Source: CAD feature listing. Evaluate the final solid. Frame: model axes, mm. Give positions to 0.01 mm unless a question says otherwise; leave off trailing zeros. Write each question's results on one line, items separated by ' | '. Start each with the question number.
Item 1: Contact query for a flat-ended pin moving along its axis: pin 1 Ø13 at (x, y) = (-143.58, -131.25) entering from +Z. Output: stop coordinate, or through.
Item 2: Line query: line 1 along X through (y, z) = (-92, 4.15); line 2 along X through (y, z) = (-92.5, 3.6); line 3 along Y through (x, z) = (-215, 0.3). Output: solid intervals per line, ascending.
Item 3: Mould query, pull axis X, two halves, no side actions, for faces 1 (the flat face through (-223.011, -76, 2)), 2 (the cylindrical face through (-189.42, -128.54, 2.54)), 3 (the flat face through (-174, -73, 0)). Classes: released by +X, released by -X, zero draft, split by the parting line, or undercut.
Item 4: Section A-A on z = 3.9. State how many separate pieces and enclosed holes the cut face has, and give its area (3 significant figures).
```python
from build123d import *

# Parameters (mm, degrees)
SKETCH2_W           = 100
SKETCH2_H           = 150
BOSS_EXTRUDE1_DEPTH = 5
SKETCH3_R           = 4.1021
CUT_EXTRUDE1_DEPTH  = 5
SKETCH6_R           = 3.2639
CUT_EXTRUDE2_DEPTH  = 269.528430204


with BuildPart() as part:
    # Sketch2 → Boss-Extrude1 (new body)
    with BuildSketch(Plane.XY):
        with Locations((-173.010889244, -74.49468588)):
            Rectangle(SKETCH2_W, SKETCH2_H)
    extrude(amount=BOSS_EXTRUDE1_DEPTH)

    # Sketch3 → Cut-Extrude1 (cut)
    with BuildSketch(Plane(origin=(0, 0, 0), x_dir=(-1, 0, 0), z_dir=(0, 0, -1))):
        with Locations((212.756022811, -54.012878845)):
            Circle(SKETCH3_R)
        with Locations((212.756022811, -94.012878845)):
            Circle(SKETCH3_R)
        with Locations((143.584758496, -18.75)):
            Circle(SKETCH3_R)
        with Locations((143.584758496, -56.25)):
            Circle(SKETCH3_R)
        with Locations((143.584758496, -93.75)):
            Circle(SKETCH3_R)
        with Locations((143.584758496, -131.25)):
            Circle(SKETCH3_R)
    extrude(amount=-CUT_EXTRUDE1_DEPTH, mode=Mode.SUBTRACT)

    # Sketch6 → Cut-Extrude2 (cut, through all)
    with BuildSketch(Plane.XY.offset(5)):
        with Locations((-187.010889244, -18.24468588)):
            Circle(SKETCH6_R)
        with Locations((-187.010889244, -55.74468588)):
            Circle(SKETCH6_R)
        with Locations((-187.010889244, -93.24468588)):
            Circle(SKETCH6_R)
        with Locations((-187.010889244, -130.74468588)):
            Circle(SKETCH6_R)
    extrude(amount=-CUT_EXTRUDE2_DEPTH, mode=Mode.SUBTRACT)


solid = part.part
```
Evaluation:
1) pin 1: stops at z = 5
2) line 1: x = -223.01 to -216.33, -209.18 to -190.03, -183.99 to -147.29, -139.87 to -123.01 | line 2: x = -223.01 to -216.57, -208.94 to -190.19, -183.83 to -147.49, -139.68 to -123.01 | line 3: y = -149.49 to -97.45, -90.58 to -57.45, -50.58 to 0.51
3) face 1: released by -X | face 2: undercut | face 3: zero draft
4) separate pieces: 1 | enclosed holes: 10 | area: 14,500 mm^2
